Could you check a few things on this drawing? It's one solid part, dimensions in mm from its lowest x, y, z. A direction names the side the tool comes from. Round coordinates to 2 decimals unless told otherwise and drop trailing zeros. Order: outer loops, then holes, each group sorted by start corner. A loop starts at its lowest first (then second) coordinate and runs counter-clockwise, first axis right, second up.
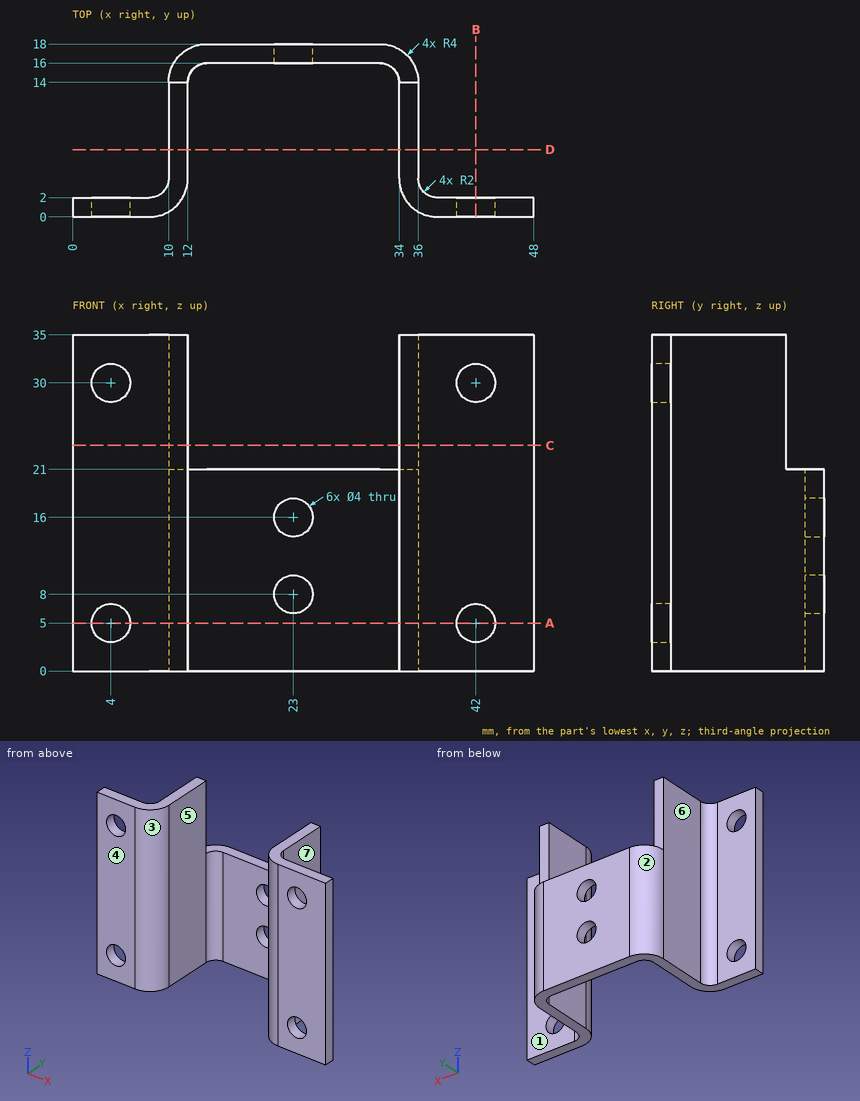
(1) I want a section at C-C, the plane z = 23.5. List the corners of the cut face in (x, y) for me.
(2) I want a section at D-D, the plane y = 7. List the corners of the cut face in (x, z) for me.
(3) On a 3-axis mill with a long thin cutter (end or side, diameter ignored), from which of +Z, -Z, +X, -X, +Y, -Y can I reach the whole of each face in a straight line? I mean the marked faces 4, 5, 6 and 7. Say none if no direction works.
(4) Please list where these lines run through material, in increasing order: probe 1 along X at (y, z) = (8.75, 3.5); probe 2 along X at (y, z) = (1.5, 5); probe 3 along Y at (x, z) = (22.5, 4).
(5) I want a section at A-A, the plane z = 5. List the corners of the cut face in (x, y) for me.
(6) If we mould it in two halves opening along X, with no side actions, what happens to the marked faces 1, 2 and 3? For each: pulls with the +X half, pulls with the -X half, needs draft (parallel to the pull), parting line crosses it, or undercut.
(7) I'm going to push flat-ended pins straight in: pin 1 Ø6 at (x, z) = (20, 7.5) entering from -Y; pin 2 Ø4.5 at (x, z) = (4, 5) entering from +Y; pin 3 Ø3 at (y, z) = (9.5, 10.5) entering from -X. Where does each tip first touch, or does it pass through?
(8) I want a section at B-B, the plane x = 42. List the corners of the cut face in (y, z) for me, plus the area to 3 significant figures.
Ans:
1. outline: (0, 0) - (8, 0) arc R4 ccw to (12, 4) - (12, 14) - (10, 14) - (10, 4) arc R2 cw to (8, 2) - (0, 2) - close; (34, 4) arc R4 ccw to (38, 0) - (48, 0) - (48, 2) - (38, 2) arc R2 cw to (36, 4) - (36, 14) - (34, 14) - close
2. outline: (10, 0) - (12, 0) - (12, 35) - (10, 35) - close; (34, 0) - (36, 0) - (36, 35) - (34, 35) - close
3. face 4: +Z, -Z, +X, -X, -Y
3. face 5: +Z, -Z, -Y
3. face 6: +Z, -Z, -X, +Y
3. face 7: +Z, -Z, +X, +Y
4. probe 1: x = 10 to 12, 34 to 36
4. probe 2: x = 0 to 2, 6 to 11.12, 34.88 to 40, 44 to 48
4. probe 3: y = 16 to 18
5. outline: (0, 0) - (2, 0) - (2, 2) - (0, 2) - close; (6, 0) - (8, 0) arc R4 ccw to (12, 4) - (12, 14) arc R2 cw to (14, 16) - (32, 16) arc R2 cw to (34, 14) - (34, 4) arc R4 ccw to (38, 0) - (40, 0) - (40, 2) - (38, 2) arc R2 cw to (36, 4) - (36, 14) arc R4 ccw to (32, 18) - (14, 18) arc R4 ccw to (10, 14) - (10, 4) arc R2 cw to (8, 2) - (6, 2) - close; (44, 0) - (48, 0) - (48, 2) - (44, 2) - close
6. face 1: needs draft
6. face 2: pulls with the -X half
6. face 3: undercut
7. pin 1: stops at y = 16
7. pin 2: stops at y = 2
7. pin 3: stops at x = 10
8. outline: (0, 0) - (2, 0) - (2, 3) - (0, 3) - close; (0, 7) - (2, 7) - (2, 28) - (0, 28) - close; (0, 32) - (2, 32) - (2, 35) - (0, 35) - close
8. area: 54.0 mm2
